```python
from build123d import *

# Parameters (mm, degrees)
SKETCH1_R           = 16.75
SKETCH1_R_2         = 12.5
BOSS_EXTRUDE1_DEPTH = 29
SKETCH2_W           = 8
SKETCH2_H           = 4
CUT_EXTRUDE2_DEPTH  = 25.5
FILLET1_R           = 2.5
FILLET2_R           = 2.5


with BuildPart() as part:
    # Sketch1 → Boss-Extrude1 (new body)
    with BuildSketch(Plane.XY):
        with Locations(Location((0, 0, 0), (0, 0, 180))):
            Circle(SKETCH1_R)
        with Locations(Location((0, 0, 0), (0, 0, 180))):
            Circle(SKETCH1_R_2, mode=Mode.SUBTRACT)
    extrude(amount=BOSS_EXTRUDE1_DEPTH)

    # Sketch2 → Cut-Extrude2 (cut)
    with BuildSketch(Plane.XY.offset(29)):
        with Locations((0, 12.5)):
            Rectangle(SKETCH2_W, SKETCH2_H)
    extrude(amount=-CUT_EXTRUDE2_DEPTH, mode=Mode.SUBTRACT)

    # Fillet1
    fillet1_edges = [part.edges().sort_by_distance(p)[0] for p in [
        (4, 13.171359641, 3.5),
    ]]
    fillet(fillet1_edges, radius=FILLET1_R)

    # Fillet2
    fillet2_edges = [part.edges().sort_by_distance(p)[0] for p in [
        (-4, 13.171359641, 3.5),
    ]]
    fillet(fillet2_edges, radius=FILLET2_R)


solid = part.part
```
Input: part model. Units: mm. Frame: model coordinates. A direction names the side the tool comes from. Coordinates: 2 decimals unless noted, no trailing zeros. Loops run counter-clockwise (first coordinate to the right, second up) from the corner with the lowest first, then second, coordinate; pieces in that order, holes last. Notation, with made-up numbers: M 47,29 L 60,29 A35 cw 60,68 Z; hole C 29,-19.5 d8. An arc over 180 degrees is marked long. Use a Markdown table: item, result. Add a question column.
1) Section C-C, the plane z = 12.75. Return the cut outline in (x, y).
2) Section D-D, the plane y = -8. Return the cut outline in (x, z), plus the area to 3 significant figures.
3) Line query: L1, parallel to Y at x = 0, z = 18.75; L2, parallel to Y at x = -7, z = 18.5; L3, parallel to X at y = 1, z = 14.75. Output: solid intervals per line, ascending. Write a range as from..to.
4) Pin query (flat end, axial travel): P1, Ø3, axis at y = 13.5, z = 21.5, coming from the +X side; P2, Ø10, axis at x = 13.5, z = 11.5, coming from the -Y side; P3, Ø5, axis at y = 13, z = 21.5, coming from the +X side. Return the tip coordinate at first contact, or that it passes through.
5) Set-up query: faces 5 (the cylindrical face through (1.627, -12.394, 14.297)), 6 (the cylindrical face through (3, 13, 4)). Return all of +Z, -Z, +X, -X, +Y, -Y with unobstructed straight access to the full face (end or side cutting, diameter ignored); none if empty.
6) Section B-B, the plane x = 0. Return the cut outline in (y, z).
7) Section A-A, the plane y = 0. Return the cut outline in (x, z).
8) Draft query along X for faces 1 (the flat face through (-4, 13, 18)), 2 (the cylindrical face through (-3, 13, 4)), 3 (the flat face through (6.3, 11.1, 0)), 4 (the cylindrical face through (-15.47, 6.42, 14.3)). Return one class per face: +X half, -X half, draft (parallel to the pull), parting line (faces both ways), or undercut.
Answer below:
| question | item | result |
|---|---|---|
| 1 | outline | C 0,0 d33.5; hole M -4,11.84 A12.5 ccw long 4,11.84 L 4,14.5 L -4,14.5 Z |
| 2 | outline | M -14.72,0 L -9.6,0 L -9.6,29 L -14.72,29 Z; M 9.6,0 L 14.72,0 L 14.72,29 L 9.6,29 Z |
| 2 | area | 296 mm2 |
| 3 | L1 | -16.75..-12.5, 14.5..16.75 |
| 3 | L2 | -15.22..-10.36, 10.36..15.22 |
| 3 | L3 | -16.72..-12.46, 12.46..16.72 |
| 4 | P1 | x = 11.69 |
| 4 | P2 | y = -14.43 |
| 4 | P3 | x = 13.05 |
| 5 | face 5 | +Z, -Z |
| 5 | face 6 | +Z |
| 6 | outline | M -16.75,0 L -12.5,0 L -12.5,29 L -16.75,29 Z; M 12.5,0 L 16.75,0 L 16.75,29 L 14.5,29 L 14.5,3.5 L 12.5,3.5 Z |
| 7 | outline | M -16.75,0 L -12.5,0 L -12.5,29 L -16.75,29 Z; M 12.5,0 L 16.75,0 L 16.75,29 L 12.5,29 Z |
| 8 | face 1 | undercut |
| 8 | face 2 | undercut |
| 8 | face 3 | draft |
| 8 | face 4 | parting line |
